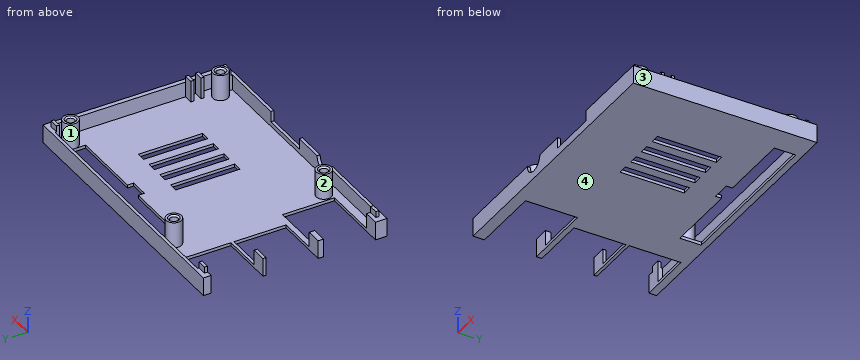
from build123d import *

# Parameters (mm, degrees)
SKETCH_W      = 3
SKETCH_H      = 21
PAD_DEPTH     = 1
SKETCH001_W   = 5
SKETCH001_H   = 1.75
SKETCH001_H_2 = 1
PAD001_DEPTH  = 5
SKETCH002_W   = 3
SKETCH002_H   = 1
PAD002_DEPTH  = 2
SKETCH003_R   = 2.5
SKETCH003_R_2 = 1.3
PAD003_DEPTH  = 8.5
SKETCH004_W   = 16
SKETCH004_H   = 3.5
POCKET_DEPTH  = 1
CHAMFER_SIZE  = 0.5
SKETCH005_W   = 3
SKETCH005_H   = 1
PAD004_DEPTH  = 7


with BuildPart() as part:
    # Sketch → Pad (new body)
    with BuildSketch(Plane.XY):
        Polygon((-45, 30), (45, 30), (45, -30), (-45, -30), (-45, -26.25), (-22, -26.25), (-22, -9.25), (-45, -9.25), (-45, -7.5), (-27, -7.5), (-27, 9.5), (-45, 9.5), (-45, 10.5), (-27, 10.5), (-27, 27.5), (-45, 27.5), align=None)
        Polygon((36.5, 21), (36.5, 28), (-16.5, 28), (-16.5, 21), (7, 21), (7, 19), (13, 19), (13, 21), align=None, mode=Mode.SUBTRACT)
        with Locations((5.5, 0)):
            Rectangle(SKETCH_W, SKETCH_H, mode=Mode.SUBTRACT)
        with Locations((11.5, 0)):
            Rectangle(SKETCH_W, SKETCH_H, mode=Mode.SUBTRACT)
        with Locations((17.5, 0)):
            Rectangle(SKETCH_W, SKETCH_H, mode=Mode.SUBTRACT)
        with Locations((23.5, 0)):
            Rectangle(SKETCH_W, SKETCH_H, mode=Mode.SUBTRACT)
    extrude(amount=PAD_DEPTH)

    # Sketch001 → Pad001 (new body)
    with BuildSketch(Plane.XY.offset(1)):
        with Locations((-42.5, -8.375)):
            Rectangle(SKETCH001_W, SKETCH001_H)
        with Locations((-42.5, 10)):
            Rectangle(SKETCH001_W, SKETCH001_H_2)
        Polygon((-45, 30), (45, 30), (45, -30), (-45, -30), (-45, -26.25), (-40, -26.25), (-40, -29), (40, -29), (40, -27.5), (43.5, -27.5), (43.5, 27.5), (40, 27.5), (40, 29), (-40, 29), (-40, 27.5), (-45, 27.5), align=None)
    extrude(amount=PAD001_DEPTH)

    # Sketch002 → Pad002 (new body)
    with BuildSketch(Plane.XY.offset(6)):
        with Locations((41.5, 28)):
            Rectangle(SKETCH002_W, SKETCH002_H)
        with Locations((-41.5, 28)):
            Rectangle(SKETCH002_W, SKETCH002_H)
        with Locations((-41.5, -28)):
            Rectangle(SKETCH002_W, SKETCH002_H)
        with Locations((41.5, -28)):
            Rectangle(SKETCH002_W, SKETCH002_H)
    extrude(amount=PAD002_DEPTH)

    # Sketch003 → Pad003 (new body)
    with BuildSketch(Plane.XY.offset(1)):
        with Locations((-19, 24.5)):
            Circle(SKETCH003_R)
        with Locations((-19, 24.5)):
            Circle(SKETCH003_R_2, mode=Mode.SUBTRACT)
        with Locations((39, 24.5)):
            Circle(SKETCH003_R)
        with Locations((39, 24.5)):
            Circle(SKETCH003_R_2, mode=Mode.SUBTRACT)
        with Locations((-19, -24.5)):
            Circle(SKETCH003_R)
        with Locations((-19, -24.5)):
            Circle(SKETCH003_R_2, mode=Mode.SUBTRACT)
        with Locations((39, -24.5)):
            Circle(SKETCH003_R)
        with Locations((39, -24.5)):
            Circle(SKETCH003_R_2, mode=Mode.SUBTRACT)
    extrude(amount=PAD003_DEPTH)

    # Sketch004 → Pocket (cut)
    with BuildSketch(Plane.XZ.offset(30)):
        with BuildLine():
            ThreePointArc((-14.5, 6), (-11, 2.5), (-7.5, 6))
            Line((-14.5, 6), (-7.5, 6))
        make_face()
        with Locations((10.5, 4.25)):
            Rectangle(SKETCH004_W, SKETCH004_H)
    extrude(amount=-POCKET_DEPTH, mode=Mode.SUBTRACT)

    # Chamfer
    chamfer_edges = [part.edges().sort_by_distance(p)[0] for p in [
        (-20.3, 24.5, 9.5),
        (37.7, 24.5, 9.5),
        (37.7, -24.5, 9.5),
        (-20.3, -24.5, 9.5),
    ]]
    chamfer(chamfer_edges, length=CHAMFER_SIZE)

    # Sketch005 → Pad004 (new body)
    with BuildSketch(Plane.XY.offset(1)):
        with Locations((42, -16.2)):
            Rectangle(SKETCH005_W, SKETCH005_H)
        with Locations((42, -19.5)):
            Rectangle(SKETCH005_W, SKETCH005_H)
    extrude(amount=PAD004_DEPTH)


solid = part.part
Read the model definition and answer for the solid it produces. Units are mm, in the model's axes. Face numbers are marked on the shaded views. Round coordinates to 2 decimals unless told otherwise and drop trailing zeros. Write each loop counter-clockwise with the first axis right and the second up, starting at its lowest first coordinate (ties: lowest second). Pieces come first, ordered by that corner, then holes. Notation, with made-up numbers: (-26.75, 83.25) - (-5.75, 83.25) arc R19 ccw to (-5.75, 98.25) - close; hole circle Ø10 at (63, 9.5). An arc over 180 degrees is marked (long way). Use a Markdown table: item, result.
(1) The part is cut by section A-A (x = -11). Write down the section's boundary in (y, z), then the cut area to 3 significant figures.
Reported:
| item | result |
|---|---|
| outline | (-30, 0) - (21, 0) - (21, 1) - (-29, 1) - (-29, 2.5) - (-30, 2.5) - close; (28, 0) - (30, 0) - (30, 6) - (29, 6) - (29, 1) - (28, 1) - close |
| area | 59.5 mm2 |
(2) Straight lines are drawn through the part: line 1 along Y through (x, z) = (39, 3.25); line 2 along Y through (x, z) = (39, 7); line 3 along X through (y, z) = (-24, 4). For each, find the intervals that lie inside material, in ascending order. Write a range as [from, to].
Reported:
| item | result |
|---|---|
| line 1 | [-30, -29], [-27, -25.8], [-23.2, -22], [22, 23.2], [25.8, 27], [29, 30] |
| line 2 | [-27, -25.8], [-23.2, -22], [22, 23.2], [25.8, 27] |
| line 3 | [-21.45, -20.2], [-17.8, -16.55], [36.55, 37.8], [40.2, 41.45], [43.5, 45] |
(3) The part is cut by section D-D (x = 39). Write down the section's boundary in (y, z), then the cut area to 3 significant figures.
Reported:
| item | result |
|---|---|
| outline | (-30, 0) - (30, 0) - (30, 6) - (29, 6) - (29, 1) - (27, 1) - (27, 9.5) - (26.3, 9.5) - (25.8, 9) - (25.8, 1) - (23.2, 1) - (23.2, 9) - (22.7, 9.5) - (22, 9.5) - (22, 1) - (-22, 1) - (-22, 9.5) - (-22.7, 9.5) - (-23.2, 9) - (-23.2, 1) - (-25.8, 1) - (-25.8, 9) - (-26.3, 9.5) - (-27, 9.5) - (-27, 1) - (-29, 1) - (-29, 6) - (-30, 6) - close |
| area | 110 mm2 |
(4) The part is cut by section C-C (x = -32). Write down the section's boundary in (y, z), then the cut area to 3 significant figures.
Reported:
| item | result |
|---|---|
| outline | (-30, 0) - (-26.25, 0) - (-26.25, 1) - (-29, 1) - (-29, 6) - (-30, 6) - close; (-9.25, 0) - (-7.5, 0) - (-7.5, 1) - (-9.25, 1) - close; (9.5, 0) - (10.5, 0) - (10.5, 1) - (9.5, 1) - close; (27.5, 0) - (30, 0) - (30, 6) - (29, 6) - (29, 1) - (27.5, 1) - close |
| area | 19.0 mm2 |
(5) The part is cut by section B-B (y = 2). Write down the section's boundary in (x, z), then the cut area to 3 significant figures.
Reported:
| item | result |
|---|---|
| outline | (-27, 0) - (4, 0) - (4, 1) - (-27, 1) - close; (7, 0) - (10, 0) - (10, 1) - (7, 1) - close; (13, 0) - (16, 0) - (16, 1) - (13, 1) - close; (19, 0) - (22, 0) - (22, 1) - (19, 1) - close; (25, 0) - (45, 0) - (45, 6) - (43.5, 6) - (43.5, 1) - (25, 1) - close |
| area | 67.5 mm2 |
(6) The mould has two halves that part along X. Classify the marked faces 1, 2, 3 and 4: released by +X, released by -X, zero draft, split by the parting line, or undercut.
Reported:
| item | result |
|---|---|
| face 1 | undercut |
| face 2 | undercut |
| face 3 | released by +X |
| face 4 | zero draft |
(7) Each of these flat-tipped pins is pushed along its axis until it touches: pin 1 Ø1.2 at (y, z) = (-18, 4.5) entering from -X; pin 2 Ø1.5 at (x, z) = (25.5, 8) entering from -Y; pin 3 Ø2 at (x, y) = (-10.5, -12) entering from +Z; pin 4 Ø5.5 at (x, z) = (3, 4) entering from -Y. Where does it stop, or does it pass through?
Reported:
| item | result |
|---|---|
| pin 1 | x = 43.5 |
| pin 2 | through |
| pin 3 | z = 1 |
| pin 4 | y = -30 |
